```python
from build123d import *

# Parameters (mm, degrees)
ESBO_O8_W                = 80
ESBO_O8_H                = 20
ESBO_O8_W_2              = 73.38
ESBO_O8_W_3              = 46.62
RESSALTO_EXTRUS_O1_DEPTH = 5
RESSALTO_EXTRUS_O2_DEPTH = 6
RESSALTO_EXTRUS_O3_DEPTH = 6
RESSALTO_EXTRUS_O4_DEPTH = 6
RESSALTO_EXTRUS_O5_DEPTH = 6
FILETE1_R                = 1
FILETE2_R                = 1


with BuildPart() as part:
    # Esboço8 → Ressalto-extrusão1 (new body)
    with BuildSketch(Plane(origin=(0, 0, 0), x_dir=(0, 0, -1), z_dir=(1, 0, 0))):
        Polygon((95.558629268, 10), (-128.441370732, 10), (-128.441370732, 42), (70.171505342, 42), (95.558629268, 42), align=None)
        with Locations((-29.821370732, 26)):
            Rectangle(ESBO_O8_W, ESBO_O8_H, mode=Mode.SUBTRACT)
        with Locations((52.868629268, 26)):
            Rectangle(ESBO_O8_W_2, ESBO_O8_H, mode=Mode.SUBTRACT)
        with Locations((-99.131370732, 26)):
            Rectangle(ESBO_O8_W_3, ESBO_O8_H, mode=Mode.SUBTRACT)
    extrude(amount=-RESSALTO_EXTRUS_O1_DEPTH)

    # Esboço9 → Ressalto-extrusão2 (add)
    with BuildSketch(Plane.XY.offset(75.821370732)):
        Polygon((-7.299581581, 42), (-5, 42), (-5, 32.104391167), (-7.299581581, 37.035859781), align=None)
    extrude(amount=-RESSALTO_EXTRUS_O2_DEPTH)

    # Esboço10 → Ressalto-extrusão3 (add)
    with BuildSketch(Plane.XY.offset(-10.178629268)):
        Polygon((-5, 32.104391167), (-5, 36), (-5, 42), (-7.299581581, 42), (-7.299581581, 37.035859781), align=None)
    extrude(amount=-RESSALTO_EXTRUS_O3_DEPTH)

    # Esboço11 → Ressalto-extrusão4 (add)
    with BuildSketch(Plane.XY.offset(128.441370732)):
        Polygon((-5, 32.104391167), (-5, 36), (-5, 42), (-7.299581581, 42), (-7.299581581, 37.035859781), align=None)
    extrude(amount=-RESSALTO_EXTRUS_O4_DEPTH)

    # Esboço12 → Ressalto-extrusão5 (add)
    with BuildSketch(Plane.XY.offset(-89.558629268)):
        Polygon((-7.299581581, 42), (-7.299581581, 37.035859781), (-5, 32.104391167), (-5, 42), align=None)
    extrude(amount=-RESSALTO_EXTRUS_O5_DEPTH)

    # Filete1
    filete1_edges = [part.edges().sort_by_distance(p)[0] for p in [
        (-6.14979079, 34.570125474, 75.821370732),
        (-6.14979079, 34.570125474, 69.821370732),
        (-7.299581581, 37.035859781, 72.821370732),
        (-7.299581581, 39.51792989, 75.821370732),
        (-7.299581581, 39.51792989, 69.821370732),
        (-7.299581581, 37.035859781, 125.441370732),
        (-7.299581581, 37.035859781, -13.178629268),
        (-3.64979079, 42, 128.441370732),
        (-7.299581581, 42, 125.441370732),
        (-6.14979079, 42, 122.441370732),
        (-5, 42, 99.131370732),
        (-6.14979079, 42, 75.821370732),
        (-7.299581581, 42, 72.821370732),
        (-6.14979079, 42, 69.821370732),
        (-5, 42, 29.821370732),
        (-6.14979079, 42, -10.178629268),
        (-7.299581581, 42, -13.178629268),
        (-6.14979079, 42, -16.178629268),
        (-5, 42, -52.868629268),
        (-6.14979079, 42, -89.558629268),
        (0, 10, 16.441370732),
        (0, 26, 128.441370732),
        (0, 42, 16.441370732),
        (0, 26, -16.178629268),
        (0, 16, -52.868629268),
        (0, 26, -89.558629268),
        (0, 36, -52.868629268),
        (0, 26, 75.821370732),
        (0, 36, 99.131370732),
        (0, 26, 122.441370732),
        (0, 16, 99.131370732),
        (0, 36, 29.821370732),
        (0, 26, 69.821370732),
        (0, 16, 29.821370732),
        (0, 26, -10.178629268),
        (-5, 24.052195584, -89.558629268),
        (-5, 16, -52.868629268),
        (-5, 24.052195584, -16.178629268),
        (-5, 32.104391167, -13.178629268),
        (-5, 24.052195584, -10.178629268),
        (-5, 16, 29.821370732),
        (-5, 24.052195584, 69.821370732),
        (-5, 32.104391167, 72.821370732),
        (-5, 24.052195584, 75.821370732),
        (-5, 16, 99.131370732),
        (-5, 24.052195584, 122.441370732),
        (-5, 32.104391167, 125.441370732),
        (-5, 21.052195584, 128.441370732),
        (-5, 10, 16.441370732),
        (-5, 36, -52.868629268),
        (-5, 36, 29.821370732),
        (-5, 36, 99.131370732),
        (-6.14979079, 34.570125474, -89.558629268),
        (-6.14979079, 34.570125474, 128.441370732),
        (-6.14979079, 34.570125474, 122.441370732),
        (-6.14979079, 34.570125474, -10.178629268),
        (-6.14979079, 34.570125474, -16.178629268),
        (-7.299581581, 39.51792989, 128.441370732),
        (-7.299581581, 39.51792989, 122.441370732),
        (-7.299581581, 39.51792989, -10.178629268),
        (-7.299581581, 39.51792989, -16.178629268),
        (-7.299581581, 42, -92.558629268),
        (-5, 32.104391167, -92.558629268),
        (-7.299581581, 37.035859781, -92.558629268),
        (-7.299581581, 39.51792989, -89.558629268),
    ]]
    fillet(filete1_edges, radius=FILETE1_R)

    # Filete2
    # the kernel refuses this fillet: 1 mm, written as the material it takes off along each edge
    with BuildSketch(Plane(origin=(-6, 31.882696504, -95.558629268), x_dir=(-0.80118997671776, -0.5984100777953153, 0), z_dir=(-0.5984100777953153, 0.80118997671776, 0))) as filete2_piece_1:
        with BuildLine():
            CenterArc((1 + FILETE2_R, FILETE2_R), FILETE2_R, 180, 90)
            Line((1, FILETE2_R), (1, 0))
            Line((1, 0), (1 + FILETE2_R, 0))
        make_face()
    revolve(axis=Axis((-6, 31.882696504, -95.558629268), (0, 0, 1)), revolution_arc=168.243887481, mode=Mode.SUBTRACT)
    with BuildSketch(Plane(origin=(-6.299581581, 37.257554444, -95.558629268), x_dir=(-1, 0, 0), z_dir=(0, 1, 0))) as filete2_piece_2:
        with BuildLine():
            CenterArc((1 - FILETE2_R, FILETE2_R), FILETE2_R, 270, 90)
            Line((1, FILETE2_R), (1, 0))
            Line((1, 0), (1 - FILETE2_R, 0))
        make_face()
    revolve(axis=Axis((-6.299581581, 37.257554444, -95.558629268), (0, 0, 1)), revolution_arc=25, mode=Mode.SUBTRACT)
    with BuildSketch(Plane(origin=(-7.205889368, 36.834936182, -95.558629268), x_dir=(0.9063077870366507, 0.4226182617406979, 0), z_dir=(0.42261826174069794, -0.9063077870366507, 0))) as filete2_piece_3:
        with BuildLine():
            CenterArc((FILETE2_R, FILETE2_R), FILETE2_R, 180, 90)
            Line((0, FILETE2_R), (0, 0))
            Line((0, 0), (FILETE2_R, 0))
        make_face()
    extrude(amount=4.997884251, mode=Mode.SUBTRACT)
    with BuildSketch(Plane(origin=(-7.299581581, 43.5, -95.558629268), x_dir=(1, 0, 0), z_dir=(0, -1, 0))) as filete2_piece_4:
        with BuildLine():
            CenterArc((FILETE2_R, FILETE2_R), FILETE2_R, 180, 90)
            Line((0, FILETE2_R), (0, 0))
            Line((0, 0), (FILETE2_R, 0))
        make_face()
    extrude(amount=6.242445556, mode=Mode.SUBTRACT)


solid = part.part
```
Here's how the part is built. I have some questions about the finished solid (model axes, mm). A direction names the side the tool comes from. Give positions to 0.01 mm unless a question says otherwise; leave off trailing zeros. Loops run counter-clockwise (first coordinate to the right, second up) from the corner with the lowest first, then second, coordinate; pieces in that order, holes last. Notation, with made-up numbers: (38.5, 69.25) -> (66.5, 69.25) arc R33 cw to (66.5, 99.25) -> close; hole circle Ø2 at (-3, -39). An arc over 180 degrees is marked (long way). Use one line per item in the form item = value. Start each with the question number.
1) Imagine slicing it at A-A (z = -19). Please give me the cut outline in (x, y).
2) Which directions (+Z, -Z, +X, -X, +Y, -Y) give clear straight access to the entire face, cutting with the end or side of a thin tool? Please do faces 1 (the face through (-5, 39, -53)), 2 (the face through (0, 37.2, 15.4)), 3 (the face through (-5, 14.5, 7.2)).
3) Please list where these lines run through material, in increasing order: line 1 along Z through (x, y) = (-1.5, 30.5); line 2 along Y through (x, z) = (-3.75, -49); line 3 along Z through (x, y) = (-4.75, 16.5).
4) Imagine slicing it at B-B (y = 26.5). Count the separate pieces of the cut face and the enclosed holes in it, then the cut area to 3 significant figures.
5) For P1, Ø12, axis at y = 35.5, z = -24.5, coming from the -X side; P2, Ø3, axis at x = -4.5, y = 22.5, coming from the +Z side, each with a flat end and sliding along its axis, tell me the tip position at first contact or that it passes through.
6) Thinking about a two-plate mould opening in Z: for faces 4 (the face through (-3, 29, 69.821)), 5 (the face through (-2, 26, -95.559)), 6 (the face through (-7.3, 39, -93)), which applies, +Z half, -Z half, draft (parallel to the pull), parting line (faces both ways), or undercut?
Check values:
q1.outline = (-5, 11) arc R1 ccw to (-4, 10) -> (-1, 10) arc R1 ccw to (0, 11) -> (0, 15) arc R1 ccw to (-1, 16) -> (-4, 16) arc R1 ccw to (-5, 15) -> close; (-5, 37) arc R1 ccw to (-4, 36) -> (-1, 36) arc R1 ccw to (0, 37) -> (0, 41) arc R1 ccw to (-1, 42) -> (-4, 42) arc R1 ccw to (-5, 41) -> close
q2.face_1 = -X, +Y, -Y
q2.face_2 = +Z, -Z, +X, +Y, -Y
q2.face_3 = +Z, -Z, -X, -Y
q3.line_1 = -95.56 to -89.56, -16.18 to -10.18, 69.82 to 75.82, 122.44 to 128.44
q3.line_2 = 10 to 16, 36 to 42
q3.line_3 = -95.56 to -89.9, -15.84 to -10.52, 70.16 to 75.48, 122.78 to 128.1
q4.separate_pieces = 4
q4.enclosed_holes = 0
q4.area = 117 mm^2
q5.P1 = -5
q5.P2 = 128.44
q6.face_4 = undercut
q6.face_5 = -Z half
q6.face_6 = draft
